Print and shaded views of the part. All mm, measured from the part's lowest x, y and z. A direction names the side the tool comes from. Round coordinates to 2 decimals unless told otherwise and drop trailing zeros. Order: outer loops, then holes, each group sorted by start corner. A loop starts at its lowest first (then second) coordinate and runs counter-clockwise, first axis right, second up. Notation, with made-up numbers: (0.5, 12.5) - (43.5, 12.5) arc R16 cw to (43.5, 30.5) - close; hole circle Ø7 at (70.5, 38). An arc over 180 degrees is marked (long way). Write item = value, one per line.
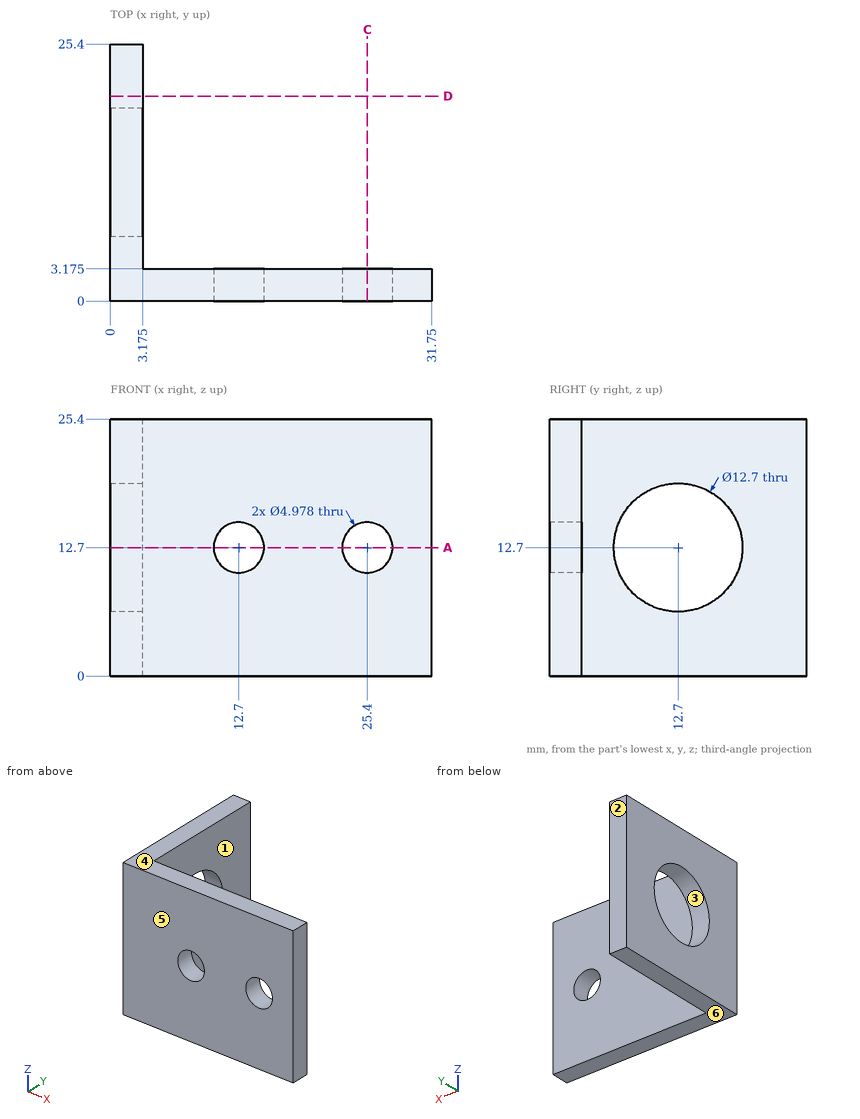
(1) Tool access for the marked faces 1 and 2: list every direction of +Z, -Z, +X, -X, +Y, -Y with a clear straight run to the whole face (end or side of a thin tool).
Solved:
face_1 = +Z, -Z, +X, +Y
face_2 = +Z, -Z, +X, -X, +Y
(2) Probe line 1 along Z through (x, y) = (12.7, 1.1); line 2 along X through (y, z) = (21.5, 1.5) (1 decimal). List the from-to ranges inside material, lowest first.
Solved:
line_1 = 0 to 10.21, 15.19 to 25.4
line_2 = 0 to 3.2
(3) Band-saw the part on C-C on x = 25.4. List the corners of the cut face in (y, z) (1 decimal).
Solved:
outline = (0, 0) - (3.2, 0) - (3.2, 10.2) - (0, 10.2) - close; (0, 15.2) - (3.2, 15.2) - (3.2, 25.4) - (0, 25.4) - close
(4) Drop flat-ended pins along their axis: pin 1 (6 mm diameter, centred on y = 10, z = 5, fed in from -X); pin 2 (11.5 mm diameter, centred on y = 12.7, z = 12.7, fed in from +X); pin 3 (3 mm diameter, centred on y = 8, z = 16, fed in from +X) (3 decimals). Give the stop position or say it passes through.
Solved:
pin_1 = 0
pin_2 = through
pin_3 = 3.175
(5) Band-saw the part on D-D on y = 20.25. List the corners of the cut face in (x, z) (1 decimal).
Solved:
outline = (0, 0) - (3.2, 0) - (3.2, 25.4) - (0, 25.4) - close
(6) Band-saw the part on A-A on z = 12.7. Count the separate pieces of the cut face and the enclosed holes in it.
Solved:
separate_pieces = 4
enclosed_holes = 0
(7) Pull direction Z, two halves, no side cores. Call the marked faces 3, 4, 5 and 6: released by +Z, released by -Z, zero draft, split by the parting line, or undercut.
Solved:
face_3 = undercut
face_4 = released by +Z
face_5 = zero draft
face_6 = released by -Z
